from build123d import *

# Parameters (mm, degrees)
SALIENTE_EXTRUIR1_DEPTH = 3


with BuildPart() as part:
    # Model → Saliente-Extruir1 (new body)
    with BuildSketch(Plane.XY):
        with BuildLine():
            Line((78.512585392, 8.480394017), (67.503193542, 8.480394017))
            Line((67.503193542, 8.480394017), (55.493801692, 8.480394017))
            Line((55.493801692, 8.480394017), (44.687089166, 3.603222324))
            Line((44.687089166, 3.603222324), (39.831918887, 14.06059302))
            Line((39.831918887, 14.06059302), (16.586059329, 8.480394017))
            Line((16.586059329, 8.480394017), (15.223673977, 21.22645362))
            ThreePointArc((15.223673977, 21.22645362), (2.983166863, 18.616670486), (-8.854222662, 14.552535688))
            ThreePointArc((-8.854222662, 14.552535688), (-10.212878112, 19.928241742), (-10.673926914, 25.453781916))
            ThreePointArc((-10.673926914, 25.453781916), (7.377127931, 35.592311556), (27.703067566, 39.527605983))
            Line((27.703067566, 39.527605983), (29.512585392, 24.480394017))
            Line((29.512585392, 24.480394017), (45.938881991, 27.30453113))
            Line((45.938881991, 27.30453113), (51.161258051, 15.555534113))
            Line((51.161258051, 15.555534113), (78.512585392, 17.480394017))
            Line((78.512585392, 17.480394017), (78.512585392, 13.980394017))
            Line((78.512585392, 13.980394017), (68.512585392, 13.980394017))
            Line((68.512585392, 13.980394017), (68.512585392, 11.980394017))
            Line((68.512585392, 11.980394017), (78.512585392, 11.980394017))
            Line((78.512585392, 11.980394017), (78.512585392, 8.480394017))
        make_face()
    extrude(amount=SALIENTE_EXTRUIR1_DEPTH)


solid = part.part
Could you check a few things on this model? Use its own coordinates, in mm. A direction names the side the tool comes from. Coordinates: 2 decimals unless noted, no trailing zeros. Write each loop counter-clockwise with the first axis right and the second up, starting at its lowest first coordinate (ties: lowest second). Pieces come first, ordered by that corner, then holes. Notation, with made-up numbers: M 43.5,60.25 L 53.5,60.25 A19 cw 53.5,85.25 Z; hole C 29,9.5 d9. An arc over 180 degrees is marked long. One line per question, with ' | ' between items.
1) Imagine slicing it at A-A, the plane y = 19.5. Write out the boundary of the cut face in (x, z), and give its area (3 significant figures).
Checks:
outline: M -10.14,0 L 6.39,0 L 6.39,3 L -10.14,3 Z; M 15.41,0 L 49.41,0 L 49.41,3 L 15.41,3 Z | area: 152 mm²
2) Imagine slicing it at B-B, the plane z = 1.2. Write out the boundary of the cut face in (x, y).
Checks:
outline: M -10.67,25.45 A33.78 ccw -8.85,14.55 A103.79 cw 15.22,21.23 L 16.59,8.48 L 39.83,14.06 L 44.69,3.6 L 55.49,8.48 L 78.51,8.48 L 78.51,11.98 L 68.51,11.98 L 68.51,13.98 L 78.51,13.98 L 78.51,17.48 L 51.16,15.56 L 45.94,27.3 L 29.51,24.48 L 27.7,39.53 A64.87 ccw Z
3) For pin 1 Ø1 at (x, z) = (64, 2) entering from +Y; pin 2 Ø1.5 at (y, z) = (24.5, 1) entering from +X; pin 3 Ø1.6 at (y, z) = (13, 2) entering from +X, each with a flat end and sliding along its axis, tell me the tip position at first contact or that it passes through.
Checks:
pin 1: y = 16.49 | pin 2: x = 47.52 | pin 3: x = 68.51
4) If we mould it in two halves opening along X, with no side actions, what happens to faces 5 (the face through (3.152, 18.663, 1.479)), 6 (the face through (-10.2, 19.85, 1.48)), 7 (the face through (78.513, 16, 1)), 8 (the face through (73, 11.98, 1))? For each: released by +X, released by -X, zero draft, split by the parting line, or undercut.
Checks:
face 5: undercut | face 6: released by -X | face 7: released by +X | face 8: zero draft
5) I need wall thicknesses on probe 1 along Y at (x, z) = (74.5, 1); probe 2 along Y at (x, z) = (72.5, 0.5); probe 3 along Y at (x, z) = (56.5, 2.55). Which ranges of each line are inside material? Lowest first, please. Write a range as [from, to].
Checks:
probe 1: [8.48, 11.98], [13.98, 17.2] | probe 2: [8.48, 11.98], [13.98, 17.06] | probe 3: [8.48, 15.93]
6) For faces 1 (the face through (64.6, 16.5, 1.5)), 2 (the face through (67, 8.48, 1)), 3 (the face through (15.914, 14.764, 1.479)), 4 (the face through (74, 13.98, 1)), which set-ups out of +Z, -Z, +X, -X, +Y, -Y let a thin tool reach every point of the face, with its end or its side?
Checks:
face 1: +Z, -Z, +Y | face 2: +Z, -Z, +X, -Y | face 3: +Z, -Z, -Y | face 4: +Z, -Z, +X
7) Imagine slicing it at D-D, the plane x = 11. Write out the boundary of the cut face in (y, z), and give its area (3 significant figures).
Checks:
outline: M 20.5,0 L 36.8,0 L 36.8,3 L 20.5,3 Z | area: 48.9 mm²
8) Imagine slicing it at C-C, the plane y = 10.5. Write out the boundary of the cut face in (x, z).
Checks:
outline: M 16.37,0 L 25,0 L 25,3 L 16.37,3 Z; M 41.49,0 L 78.51,0 L 78.51,3 L 41.49,3 Z
